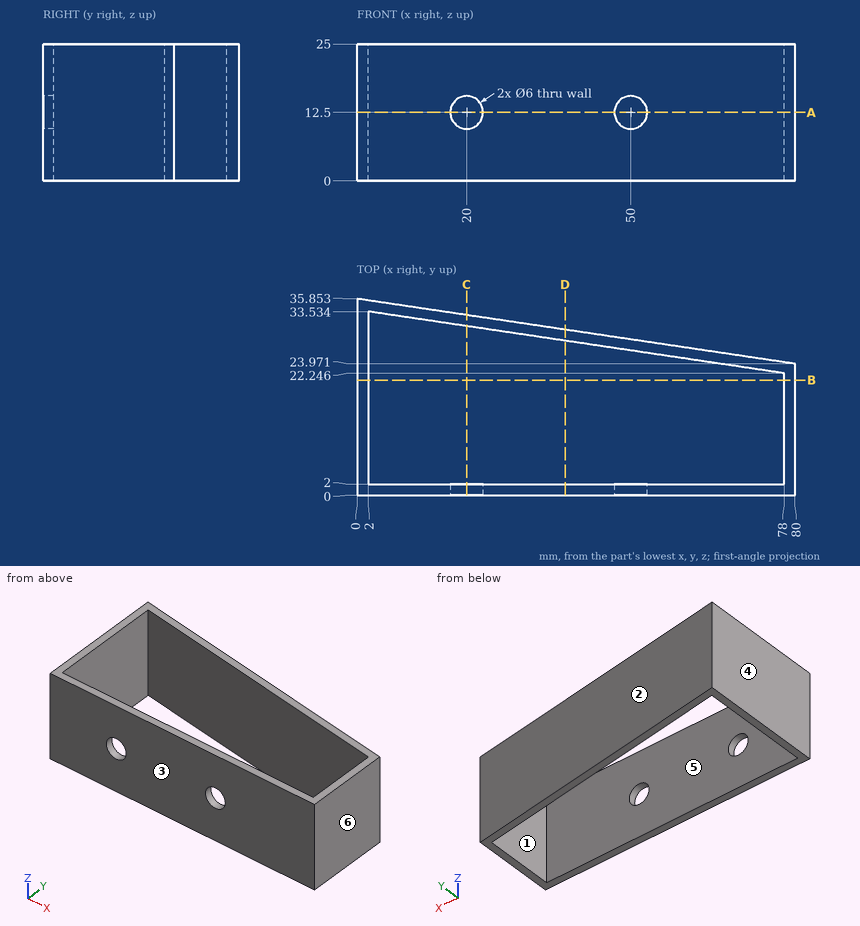
Print and shaded views of the part. All mm, measured from the part's lowest x, y and z. A direction names the side the tool comes from. Give positions to 0.01 mm unless a question says otherwise; leave off trailing zeros. Loops run counter-clockwise (first coordinate to the right, second up) from the corner with the lowest first, then second, coordinate; pieces in that order, holes last.
1) Tool access for the marked faces 1 and 2: list every direction of +Z, -Z, +X, -X, +Y, -Y with a clear straight run to the whole face (end or side of a thin tool).
2) Saw through at A-A (z = 12.5). Write the cut outline in (x, y) (1 decimal).
3) Saw through at B-B (y = 21). Write the cut outline in (x, z).
4) Saw through at D-D (x = 38). Write the cut outline in (y, z).
5) Saw through at C-C (x = 20). Write the cut outline in (y, z).
6) Flat gauge pins, fed straight in: pin 1 Ø5 at (x, z) = (50, 12.5) entering from -Y; pin 2 Ø3.5 at (x, z) = (20, 12.5) entering from -Y. Where does each tip first touch, or does it go through?
7) Wall check: line 1 (X direction, y = 20.5, z = 22); line 2 (Z direction, x = 50, y = 0.5); line 3 (Y direction, x = 5.5, z = 12) (1 decimal). Give the ranges that are in metal, low to high.
8) Pull direction X, two halves, no side cores. Call the marked faces 3, 4, 5 and 6: +X half, -X half, draft (parallel to the pull), parting line (faces both ways), or undercut.
Answer block:
1. face 1: +Z, -Z
1. face 2: +Z, -Z, +X, +Y
2. outline: (0, 0) - (17, 0) - (17, 2) - (2, 2) - (2, 33.5) - (78, 22.2) - (78, 2) - (53, 2) - (53, 0) - (80, 0) - (80, 24) - (0, 35.9) - close; (23, 0) - (47, 0) - (47, 2) - (23, 2) - close
3. outline: (0, 0) - (2, 0) - (2, 25) - (0, 25) - close; (78, 0) - (80, 0) - (80, 25) - (78, 25) - close
4. outline: (0, 0) - (2, 0) - (2, 25) - (0, 25) - close; (28.19, 0) - (30.21, 0) - (30.21, 25) - (28.19, 25) - close
5. outline: (0, 0) - (2, 0) - (2, 9.5) - (0, 9.5) - close; (0, 15.5) - (2, 15.5) - (2, 25) - (0, 25) - close; (30.86, 0) - (32.88, 0) - (32.88, 25) - (30.86, 25) - close
6. pin 1: stops at y = 26.03
6. pin 2: stops at y = 30.6
7. line 1: x = 0 to 2, 78 to 80
7. line 2: z = 0 to 9.5, 15.5 to 25
7. line 3: y = 0 to 2, 33 to 35
8. face 3: draft
8. face 4: -X half
8. face 5: undercut
8. face 6: +X half
